from build123d import *

# Parameters (mm, degrees)
BOSS_EXTRUDE1_DEPTH = 7.9248
SKETCH1_R           = 15.113
SKETCH1_R_2         = 4.7625
CUT_EXTRUDE1_DEPTH  = 80.272040778
BOSS_EXTRUDE2_DEPTH = 101.6
BOSS_EXTRUDE3_START = 50.8
BOSS_EXTRUDE3_DEPTH = 50.8


with BuildPart() as part:
    # Sketch3 → Boss-Extrude1 (new body)
    with BuildSketch(Plane.XY):
        with BuildLine():
            Line((-64.234613185, 11.323473258), (-41.773518083, 22.268986661))
            ThreePointArc((-41.773518083, 22.268986661), (-35.255720627, 22.619332528), (-30.461132459, 18.190297621))
            Line((-30.461132459, 18.190297621), (-18.440189358, -8.351633097))
            ThreePointArc((-18.440189358, -8.351633097), (0, -20.243279352), (18.440189358, -8.351633097))
            Line((18.440189358, -8.351633097), (30.461132459, 18.190297621))
            ThreePointArc((30.461132459, 18.190297621), (35.255720627, 22.619332528), (41.773518083, 22.268986661))
            Line((41.773518083, 22.268986661), (64.234613185, 11.323473258))
            ThreePointArc((64.234613185, 11.323473258), (69.246925134, 3.525173307), (64.633248189, -4.515394972))
            Line((64.633248189, -4.515394972), (8.109165467, -35.67188883))
            ThreePointArc((8.109165467, -35.67188883), (0, -37.758787862), (-8.109165467, -35.67188883))
            Line((-8.109165467, -35.67188883), (-64.633248189, -4.515394972))
            ThreePointArc((-64.633248189, -4.515394972), (-69.246925134, 3.525173307), (-64.234613185, 11.323473258))
        make_face()
    extrude(amount=BOSS_EXTRUDE1_DEPTH)

    # Sketch1 → Cut-Extrude1 (cut, through all)
    with BuildSketch(Plane.XY):
        Circle(SKETCH1_R)
        with Locations((-60.325, 3.300624961)):
            Circle(SKETCH1_R_2)
        with Locations((-38.1, 14.730624961)):
            Circle(SKETCH1_R_2)
        with Locations(Location((38.1, 14.730624961, 0), (0, 0, 180))):
            Circle(SKETCH1_R_2)
        with Locations(Location((60.325, 3.300624961, 0), (0, 0, 180))):
            Circle(SKETCH1_R_2)
    extrude(amount=CUT_EXTRUDE1_DEPTH, mode=Mode.SUBTRACT)

    # Sketch4 → Boss-Extrude2 (add)
    with BuildSketch(Plane.XY.offset(7.9248)):
        with BuildLine():
            ThreePointArc((-40.926635767, 27.63434288), (-20.582852086, 30.953683993), (0, 32.064431449))
            ThreePointArc((0, 32.064431449), (20.582852086, 30.953683993), (40.926635767, 27.63434288))
            ThreePointArc((40.926635767, 27.63434288), (51.23189196, 13.299115463), (38.080011359, 1.520954021))
            ThreePointArc((38.080011359, 1.520954021), (26.188891906, -1.306064402), (16.866232202, -9.210415804))
            ThreePointArc((16.866232202, -9.210415804), (9.454365502, -15.499494869), (0, -17.758533696))
            ThreePointArc((0, -17.758533696), (-9.454365502, -15.499494869), (-16.866232202, -9.210415804))
            ThreePointArc((-16.866232202, -9.210415804), (-26.188891906, -1.306064402), (-38.080011359, 1.520954021))
            ThreePointArc((-38.080011359, 1.520954021), (-51.23189196, 13.299115463), (-40.926635767, 27.63434288))
        make_face()
    extrude(amount=BOSS_EXTRUDE2_DEPTH)

    # Sketch5 → Boss-Extrude3 (add)
    with BuildSketch(Plane(origin=(0, 0, 7.9248), x_dir=(-1, 0, 0), z_dir=(0, 0, -1)).offset(BOSS_EXTRUDE3_START)):
        with BuildLine():
            ThreePointArc((-47.327995259, 26.116255836), (0, 32.064431449), (47.327995259, 26.116255836))
            ThreePointArc((47.327995259, 26.116255836), (49.920381816, 21.745535091), (45.549661071, 19.153148533))
            ThreePointArc((45.549661071, 19.153148533), (0, 24.877823363), (-45.549661071, 19.153148533))
            ThreePointArc((-45.549661071, 19.153148533), (-49.920381816, 21.745535091), (-47.327995259, 26.116255836))
        make_face()
    extrude(amount=-BOSS_EXTRUDE3_DEPTH)


solid = part.part
Work out the finished part from the listing and answer in its coordinate system (mm). A direction names the side the tool comes from. Round coordinates to 2 decimals unless told otherwise and drop trailing zeros. Write each loop counter-clockwise with the first axis right and the second up, starting at its lowest first coordinate (ties: lowest second). Pieces come first, ordered by that corner, then holes.
1) A cutting plane is placed at D-D (z = -26). Give the vertices of the cut face in (x, y), plus the area to 3 significant figures.
2) A cutting plane is placed at B-B (y = -12). Give the vertices of the cut face in (x, z).
3) A tool of negligible diameter and unlimited length cuts with its end or side. For faces 4 (the flat face through (-1, 26, -42.875)), 5 (the cylindrical face through (-42.858, 14.94, 3.907)), 6 (the flat face through (-48, 25, 7.925)), from which of +Z, -Z, +X, -X, +Y, -Y can it reach the whole face along a straight path? Write none if from no direction.
4) A cutting plane is placed at A-A (x = 60). Give the vertices of the cut face in (y, z).
5) Straight lines are drawn through the part: line 1 (Z direction, x = 15, y = -15.5); line 2 (X direction, y = 11.5, z = 46); line 3 (Y direction, x = 38.1, z = 4). For each, find the intervals that lie inside material, in ascending order.
6) The mould has two halves that part along Y. Classify faces 1 (the flat face through (0, 9, 7.925)), 2 (the flat face through (0, -22, 7.925)), 3 (the cylindrical face through (-26.04, -1.38, 58.01)): pulls with the +Y half, pulls with the -Y half, needs draft (parallel to the pull), parting line crosses it, or undercut.
7) A cutting plane is placed at C-C (z = 29). Give the vertices of the cut face in (x, y).
8) Given pin 1 Ø21.5 at (x, y) = (-1, -6.5) entering from -Z; pin 2 Ø12 at (x, z) = (-20, 84) entering from +Y; pin 3 Ø1.5 at (y, z) = (16, 85.5) entering from -X, each flat-ended and moving along its own axis, determine where each tip first touches the part or whether it passes through.
Completed:
1. outline: (-47.33, 26.12) arc R3.59 ccw to (-45.55, 19.15) arc R184.08 cw to (45.55, 19.15) arc R3.59 ccw to (47.33, 26.12) arc R191.26 ccw to start
1. area: 715 mm2
2. outline: (-51.05, 0) - (-16.3, 0) - (-16.3, 7.92) - (-51.05, 7.92) - close; (-14.41, 7.92) - (14.41, 7.92) - (14.41, 109.52) - (-14.41, 109.52) - close; (16.3, 0) - (51.05, 0) - (51.05, 7.92) - (16.3, 7.92) - close
3. face 4: -Z, +X, -X, +Y, -Y
3. face 5: -Z
3. face 6: +Z, -X, +Y
4. outline: (-7.07, 0) - (-1.45, 0) - (-1.45, 7.92) - (-7.07, 7.92) - close; (8.05, 0) - (13.39, 0) - (13.39, 7.92) - (8.05, 7.92) - close
5. line 1: z = 0 to 7.92
5. line 2: x = -50.91 to 50.91
5. line 3: y = -19.14 to 9.97, 19.49 to 28.23
6. face 1: undercut
6. face 2: needs draft
6. face 3: pulls with the -Y half
7. outline: (-40.93, 27.63) arc R13.21 ccw to (-38.08, 1.52) arc R26.25 cw to (-16.87, -9.21) arc R20.91 ccw to (16.87, -9.21) arc R26.25 cw to (38.08, 1.52) arc R13.21 ccw to (40.93, 27.63) arc R191.26 ccw to start
8. pin 1: stops at z = 7.92
8. pin 2: stops at y = 31.55
8. pin 3: stops at x = -51.3
